Could you check a few things on this model? Use its own coordinates, in mm. A direction names the side the tool comes from. Give positions to 0.01 mm unless a question says otherwise; leave off trailing zeros. Loops run counter-clockwise (first coordinate to the right, second up) from the corner with the lowest first, then second, coordinate; pieces in that order, holes last. Notation, with made-up numbers: (80, -26) -> (126, -26) arc R30 ccw to (126, 4) -> close; hole circle Ø10 at (24.25, 55). An arc over 180 degrees is marked (long way). Put each result on its own line as item: value.
Autodesk Inventor part; units mm, degrees
ref_plane "Work Plane1" through (-254, 0, 0) normal (1, 0, 0) x (0, 1, 0)
ref_plane "YZ Plane" through (0, 0, 0) normal (1, 0, 0) x (0, 1, 0)
ref_plane "XZ Plane" through (0, 0, 0) normal (0, 1, 0) x (-1, 0, 0)
sketch "Sketch1" plane through (0, 0, 0) normal (0, 0, 1) x (1, 0, 0)
  line L0 (-254, 0) -> (0, 0)
  line L1 (0, 0) -> (0, 254)
  line L2 (-215.5261, 0) -> (0, 215.5261)
  dimension "d0" = 254
  dimension "d1" = 254
  dimension "d2" = 90
  dimension "d5" = 152.4
  dimension "d6" = 45
ref_plane "Work Plane1" through (-254, 0, 0) normal (1, 0, 0) x (0, 1, 0)
sketch "Sketch2" plane through (-254, 0, 0) normal (1, 0, 0) x (0, 1, 0)
  circle A0 centre (0, 0) radius 19.05
  dimension "d3" = 38.1
sweep "Sweep1" add profiles "Sketch2" path "Sketch1" path curves L0 L1
extrude "Extrusion1" add sketch "Sketch1" against normal blind 3.175
properties part number "corner_prop"
1. I need wall thicknesses on line 1 (Z direction, x = -1.5, y = 173); line 2 (Z direction, x = -51.5, y = 125.5) (3 decimals); line 3 (X direction, y = 188, z = 1). Which ranges of each line are inside material? Lowest first, please.
Recorded:
line 1: z = -18.99 to 18.99
line 2: z = -3.175 to 0
line 3: x = -19.02 to 19.02
2. I'm going to push flat-ended pins straight in: pin 1 (3 mm diameter, centred on y = 132.5, z = -12.5, fed in from +X); pin 2 (3 mm diameter, centred on x = -80.5, z = 8.5, fed in from +Y); pin 3 (3 mm diameter, centred on y = 129.5, z = -4.5, fed in from -X). Where does each tip first touch, or does it pass through?
Recorded:
pin 1: stops at x = 15.55
pin 2: stops at y = 17.72
pin 3: stops at x = -86.73
3. If we section it at C-C (z = -8): List the corners of the cut face in (x, y) for me.
Recorded:
outline: (-254, -17.29) -> (17.29, -17.29) -> (17.29, 254) -> (-17.29, 254) -> (-17.29, 17.29) -> (-254, 17.29) -> close
4. If we section it at A-A (x = -228.5): List the corners of the cut face in (y, z) for me.
Recorded:
outline: circle Ø38.1 at (0, 0)
5. If we section it at D-D (x = -171): List the corners of the cut face in (y, z) for me (3 decimals), then the cut area to 3 significant figures.
Recorded:
outline: (18.784, -3.175) -> (44.526, -3.175) -> (44.526, 0) -> (19.05, 0) arc R19.05 ccw (long way) to start
area: 1,220 mm^2
6. For faces 1 (the face through (-69, 69, -3.175)), 2 (the face through (-70, 70, 0)), 3 (the face through (19.03, 119.39, 0.84)), which set-ups out of +Z, -Z, +X, -X, +Y, -Y let a thin tool reach every point of the face, with its end or its side?
Recorded:
face 1: -Z, -X, +Y
face 2: +Z, -X, +Y
face 3: +Y
7. If we section it at B-B (y = 155): List the corners of the cut face in (x, z) for me (3 decimals), then the cut area to 3 significant figures.
Recorded:
outline: (-60.526, -3.175) -> (-18.784, -3.175) arc R19.05 ccw (long way) to (-19.05, 0) -> (-60.526, 0) -> close
area: 1,270 mm^2
